Here's how the part is built. I have some questions about the finished solid (model axes, mm). Round coordinates to 2 decimals unless told otherwise and drop trailing zeros. Loops run counter-clockwise (first coordinate to the right, second up) from the corner with the lowest first, then second, coordinate; pieces in that order, holes last. Notation, with made-up numbers: M 14,62.25 L 54,62.25 A20 ccw 54,96.25 Z; hole C 33.5,-15.5 d10. An arc over 180 degrees is marked long. Write each question's results on one line, items separated by ' | '. Start each with the question number.
```python
from build123d import *

# Parameters (mm, degrees)
SKETCH2_W           = 100
SKETCH2_H           = 20
BOSS_EXTRUDE1_DEPTH = 3
SKETCH3_R           = 5
CUT_EXTRUDE1_DEPTH  = 103.02450686
SKETCH4_R           = 5
CUT_EXTRUDE2_DEPTH  = 103.02450686
FILLET1_R           = 10
FILLET2_R           = 10


with BuildPart() as part:
    # Sketch2 → Boss-Extrude1 (new body)
    with BuildSketch(Plane(origin=(0, 0, 0), x_dir=(1, 0, 0), z_dir=(0, 1, 0))):
        with Locations((50, 10)):
            Rectangle(SKETCH2_W, SKETCH2_H)
    extrude(amount=BOSS_EXTRUDE1_DEPTH)

    # Sketch3 → Cut-Extrude1 (cut, through all)
    with BuildSketch(Plane(origin=(0, 3, 0), x_dir=(1, 0, 0), z_dir=(0, 1, 0))):
        with Locations(Location((9, 10, 0), (0, 0, 270))):
            Circle(SKETCH3_R)
    extrude(amount=-CUT_EXTRUDE1_DEPTH, mode=Mode.SUBTRACT)

    # Sketch4 → Cut-Extrude2 (cut, through all)
    with BuildSketch(Plane(origin=(0, 3, 0), x_dir=(1, 0, 0), z_dir=(0, 1, 0))):
        with Locations(Location((91, 10, 0), (0, 0, 270))):
            Circle(SKETCH4_R)
    extrude(amount=-CUT_EXTRUDE2_DEPTH, mode=Mode.SUBTRACT)

    # Fillet1
    fillet1_edges = [part.edges().sort_by_distance(p)[0] for p in [
        (0, 1.5, -20),
        (0, 1.5, 0),
    ]]
    fillet(fillet1_edges, radius=FILLET1_R - 0.0001)  # a hair under: the kernel refuses the full size

    # Fillet2
    fillet2_edges = [part.edges().sort_by_distance(p)[0] for p in [
        (100, 1.5, -20),
        (100, 1.5, 0),
    ]]
    fillet(fillet2_edges, radius=FILLET2_R - 0.0001)  # a hair under: the kernel refuses the full size


solid = part.part
```
1. I want a section at C-C on x = 6. List the corners of the cut face in (y, z) for me.
2. I want a section at A-A on y = 2.3. Count the separate pieces of the cut face and the enclosed holes in it, plus the area to 3 significant figures.
3. For pin 1 (5 mm diameter, centred on x = 10.5, z = -9.5, fed in from -Y), with a flat end and sliding along its axis, tell me the tip position at first contact or that it passes through.
4. I want a section at D-D on z = -13.75. List the corners of the cut face in (x, y) for me.
5. I want a section at B-B on z = -6. List the corners of the cut face in (x, y) for me, plus the area to 3 significant figures.
6. If we mould it in two halves opening along X, with no side actions, what happens to faces 1 (the face through (10.5, 1.52, -5.23)), 2 (the face through (49, 1, 0)), 3 (the face through (96.99, 1.52, -17.15))? For each: released by +X, released by -X, zero draft, split by the parting line, or undercut.
7. I need wall thicknesses on line 1 along X through (y, z) = (1.4, -10); line 2 along X through (y, z) = (2.3, -8.75); line 3 along Z through (x, y) = (92, 1.5). Which ranges of each line are inside material? Lowest first, please.
Outcome:
1) outline: M 0,-19.17 L 3,-19.17 L 3,-14 L 0,-14 Z; M 0,-6 L 3,-6 L 3,-0.83 L 0,-0.83 Z
2) separate pieces: 1 | enclosed holes: 2 | area: 1,760 mm2
3) pin 1: through
4) outline: M 0.73,0 L 5.69,0 L 5.69,3 L 0.73,3 Z; M 12.31,0 L 87.69,0 L 87.69,3 L 12.31,3 Z; M 94.31,0 L 99.27,0 L 99.27,3 L 94.31,3 Z
5) outline: M 0.83,0 L 6,0 L 6,3 L 0.83,3 Z; M 12,0 L 88,0 L 88,3 L 12,3 Z; M 94,0 L 99.17,0 L 99.17,3 L 94,3 Z | area: 259 mm2
6) face 1: undercut | face 2: zero draft | face 3: released by +X
7) line 1: 0 to 4, 14 to 86, 96 to 100 | line 2: 0.08 to 4.16, 13.84 to 86.16, 95.84 to 99.92 | line 3: -19.8 to -14.9, -5.1 to -0.2
